Here's how the part is built. I have some questions about the finished solid (model axes, mm). Coordinates: 2 decimals unless noted, no trailing zeros. Order: outer loops, then holes, each group sorted by start corner. A loop starts at its lowest first (then second) coordinate and runs counter-clockwise, first axis right, second up. Notation, with made-up numbers: (-31.5, 29) -> (-6.5, 29) arc R34 cw to (-6.5, 59) -> close; hole circle Ø1 at (89, 86.5). An arc over 180 degrees is marked (long way). One line per item, written item: value. Start each with the question number.
```python
from build123d import *

# Parameters (mm, degrees)
CYLINDER001_R     = 4
CYLINDER001_DEPTH = 12
CYLINDER_R        = 6.12
CYLINDER_DEPTH    = 12
CHAMFER_SIZE      = 1.9


with BuildPart() as cilindro001:
    # Cylinder001 → Cylinder001 (new body)
    with BuildSketch(Plane.XY):
        Circle(CYLINDER001_R)
    extrude(amount=CYLINDER001_DEPTH)


with BuildPart() as chamfer_body:
    # Cylinder → Cylinder (new body)
    with BuildSketch(Plane.XY):
        Circle(CYLINDER_R)
    extrude(amount=CYLINDER_DEPTH)

    # Cut: cut Cilindro001
    add(cilindro001.part, mode=Mode.SUBTRACT)

    # Chamfer
    chamfer_edges = [chamfer_body.edges().sort_by_distance(p)[0] for p in [
        (-4, 0, 12),
    ]]
    chamfer(chamfer_edges, length=CHAMFER_SIZE)


solid = chamfer_body.part
```
Q1. Imagine slicing it at D-D (z = 10.75). Write out the boundary of the cut face in (x, y).
Q2. Imagine slicing it at C-C (z = 8). Write out the boundary of the cut face in (x, y), plus the area to 3 significant figures.
Q3. Imagine slicing it at A-A (y = 0). Write out the boundary of the cut face in (x, z).
Q4. I need wall thicknesses on line 1 (Y direction, x = 0, z = 7); line 2 (Y direction, x = -1.75, z = 5.5); line 3 (X direction, y = -4, z = 11). Which ranges of each line are inside material? Lowest first, please.
Q5. For P1, Ø2, axis at y = -4, z = 7.5, coming from the +X side; P2, Ø1, axis at y = 3, z = 4.5, coming from the +X side; P3, Ø1, axis at y = -3.5, z = 5, coming from the -X side, each with a flat end and sliding along its axis, tell me the tip position at first contact or that it passes through.
Q6. If we mould it in two halves opening along X, with no side actions, what happens to faces 1 (the face through (1.3, -4, 0)), 2 (the face through (-4.86, -3.72, 5.92)), 3 (the face through (-0.867, -3.905, 4.979))? For each: +X half, -X half, draft (parallel to the pull), parting line (faces both ways), or undercut.
Completed:
1. outline: circle Ø12.24 at (0, 0); hole circle Ø9.3 at (0, 0)
2. outline: circle Ø12.24 at (0, 0); hole circle Ø8 at (0, 0)
2. area: 67.4 mm2
3. outline: (-6.12, 0) -> (-4, 0) -> (-4, 10.1) -> (-5.9, 12) -> (-6.12, 12) -> close; (4, 0) -> (6.12, 0) -> (6.12, 12) -> (5.9, 12) -> (4, 10.1) -> close
4. line 1: y = -6.12 to -4, 4 to 6.12
4. line 2: y = -5.86 to -3.6, 3.6 to 5.86
4. line 3: x = -4.63 to -2.83, 2.83 to 4.63
5. P1: stops at x = 5.33
5. P2: stops at x = 5.59
5. P3: stops at x = -5.33
6. face 1: draft
6. face 2: parting line
6. face 3: undercut
